from build123d import *

# Parameters (mm, degrees)
SKETCH1_R           = 1.1938
BOSS_EXTRUDE1_DEPTH = 1.5875
SKETCH2_R           = 1.1938
BOSS_EXTRUDE2_DEPTH = 1.5875
BOSS_EXTRUDE3_DEPTH = 3.175
BOSS_EXTRUDE4_DEPTH = 3.175
SKETCH5_W           = 3.656154394
SKETCH5_H           = 41.933387184
CUT_EXTRUDE1_DEPTH  = 78.415745756


with BuildPart() as part:
    # Sketch1 → Boss-Extrude1 (new, symmetric)
    with BuildSketch(Plane(origin=(0, 0, 0), x_dir=(1, 0, 0), z_dir=(0, 1, 0))):
        with BuildLine():
            Line((-40.9956, 2.7686), (40.9956, 2.7686))
            ThreePointArc((40.9956, 2.7686), (43.7642, 0), (40.9956, -2.7686))
            Line((40.9956, -2.7686), (-40.9956, -2.7686))
            ThreePointArc((-40.9956, -2.7686), (-43.7642, 0), (-40.9956, 2.7686))
        make_face()
        with Locations(Location((-40.9956, 0, 0), (0, 0, 270))):
            Circle(SKETCH1_R, mode=Mode.SUBTRACT)
        with Locations(Location((40.9956, 0, 0), (0, 0, 270))):
            Circle(SKETCH1_R, mode=Mode.SUBTRACT)
    extrude(amount=BOSS_EXTRUDE1_DEPTH, both=True)



with BuildPart() as body_2:
    # Sketch2 → Boss-Extrude2 (new, symmetric)
    with BuildSketch(Plane(origin=(0, 0, 0), x_dir=(1, 0, 0), z_dir=(0, 1, 0))):
        with BuildLine():
            Line((-40.9956, -58.2422), (40.9956, -58.2422))
            ThreePointArc((40.9956, -58.2422), (43.7642, -61.0108), (40.9956, -63.7794))
            Line((40.9956, -63.7794), (-40.9956, -63.7794))
            ThreePointArc((-40.9956, -63.7794), (-43.7642, -61.0108), (-40.9956, -58.2422))
        make_face()
        with Locations(Location((-40.9956, -61.0108, 0), (0, 0, 270))):
            Circle(SKETCH2_R, mode=Mode.SUBTRACT)
        with Locations(Location((40.9956, -61.0108, 0), (0, 0, 270))):
            Circle(SKETCH2_R, mode=Mode.SUBTRACT)
    extrude(amount=BOSS_EXTRUDE2_DEPTH, both=True)


with BuildPart() as part_1:
    add(part.part)

    add(body_2.part)  # Boss-Extrude3 merges body 2
    # Sketch3 → Boss-Extrude3 (add)
    with BuildSketch(Plane(origin=(0, 1.5875, 0), x_dir=(1, 0, 0), z_dir=(0, 1, 0))):
        with BuildLine():
            ThreePointArc((-40.9956, -2.7686), (-42.953295834, -1.957695834), (-43.7642, 0))
            Line((-43.7642, 0), (-43.7642, -61.0108))
            ThreePointArc((-43.7642, -61.0108), (-42.953295834, -59.053104166), (-40.9956, -58.2422))
            Line((-40.9956, -58.2422), (-36.444722592, -58.2422))
            Line((-36.444722592, -58.2422), (-36.444722592, -2.7686))
            Line((-36.444722592, -2.7686), (-40.9956, -2.7686))
        make_face()
    extrude(amount=-BOSS_EXTRUDE3_DEPTH)

    # Sketch4 → Boss-Extrude4 (add)
    with BuildSketch(Plane(origin=(0, 1.5875, 0), x_dir=(1, 0, 0), z_dir=(0, 1, 0))):
        with BuildLine():
            ThreePointArc((40.9956, -58.2422), (42.953295834, -59.053104166), (43.7642, -61.0108))
            Line((43.7642, -61.0108), (43.7642, -12.9794))
            Line((43.7642, -12.9794), (34.8742, -12.9794))
            Line((34.8742, -12.9794), (34.8742, -58.2422))
            Line((34.8742, -58.2422), (40.9956, -58.2422))
        make_face()
    extrude(amount=-BOSS_EXTRUDE4_DEPTH)

    # Sketch5 → Cut-Extrude1 (cut, through all)
    with BuildSketch(Plane(origin=(0, 1.5875, 0), x_dir=(1, 0, 0), z_dir=(0, 1, 0))):
        with Locations((41.936122803, -33.946093592)):
            Rectangle(SKETCH5_W, SKETCH5_H)
    extrude(amount=-CUT_EXTRUDE1_DEPTH, mode=Mode.SUBTRACT)


solid = part_1.part
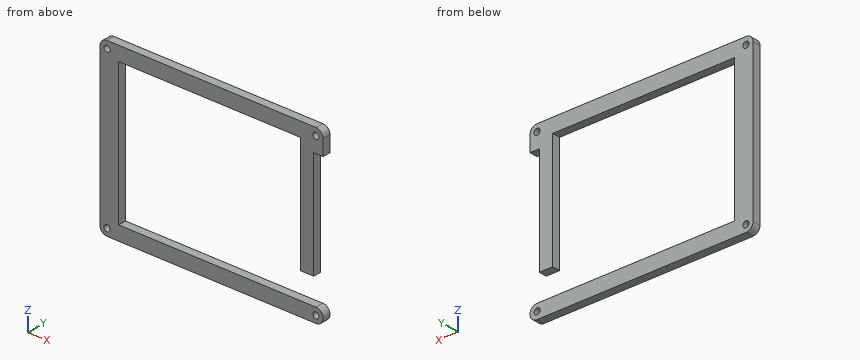
Could you check a few things on this model? Use its own coordinates, in mm. Give positions to 0.01 mm unless a question says otherwise; leave off trailing zeros. Loops run counter-clockwise (first coordinate to the right, second up) from the corner with the lowest first, then second, coordinate; pieces in that order, holes last. Notation, with made-up numbers: (89, -4) -> (144, -4) arc R27 ccw to (144, 30) -> close; hole circle Ø5 at (-16.75, 45). An arc over 180 degrees is marked (long way). Return JSON: item names as keys, results as strings.
Item 1: If we section it at B-B on y = -0.4: List the corners of the cut face in (x, z) for me.
Geometry results:
{"outline": "(-43.76, 0) arc R2.77 ccw to (-41, -2.77) -> (41, -2.77) arc R2.77 ccw to (41, 2.77) -> (-36.44, 2.77) -> (-36.44, 58.24) -> (34.87, 58.24) -> (34.87, 12.98) -> (40.11, 12.98) -> (40.11, 54.91) -> (43.76, 54.91) -> (43.76, 61.01) arc R2.77 ccw to (41, 63.78) -> (-41, 63.78) arc R2.77 ccw to (-43.76, 61.01) -> close; hole circle Ø2.39 at (-41, 0); hole circle Ø2.39 at (-41, 61.01); hole circle Ø2.39 at (41, 0); hole circle Ø2.39 at (41, 61.01)"}
Item 2: I'm going to push flat-ended pins straight in: pin 1 (1 mm diameter, centred on y = -0.5, z = 32.5, fed in from +X); pin 2 (1.6 mm diameter, centred on x = 42, y = 0, fed in from -Z). Where does each tip first touch, or does it pass through?
Geometry results:
{"pin 1": "stops at x = 40.11", "pin 2": "stops at z = -2.76"}
Item 3: I need wall thicknesses on L1, parallel to X at y = 0.7, z = 0; L2, parallel to X at y = 1.45, z = 50.5; L3, parallel to Z at x = -15.5, y = -1.45. Which ranges of each line are inside material? Lowest first, please. Write a range as from..to.
Geometry results:
{"L1": "x = -43.76..-42.19, -39.8..39.8, 42.19..43.76", "L2": "x = -43.76..-36.44, 34.87..40.11", "L3": "z = -2.77..2.77, 58.24..63.78"}
Item 4: If we section it at C-C on x = -15: List the corners of the cut face in (y, z) for me.
Geometry results:
{"outline": "(-1.59, -2.77) -> (1.59, -2.77) -> (1.59, 2.77) -> (-1.59, 2.77) -> close; (-1.59, 58.24) -> (1.59, 58.24) -> (1.59, 63.78) -> (-1.59, 63.78) -> close"}
Item 5: If we section it at A-A on z = 42.5: List the corners of the cut face in (x, y) for me, plus the area to 3 significant figures.
Geometry results:
{"outline": "(-43.76, -1.59) -> (-36.44, -1.59) -> (-36.44, 1.59) -> (-43.76, 1.59) -> close; (34.87, -1.59) -> (40.11, -1.59) -> (40.11, 1.59) -> (34.87, 1.59) -> close", "area": "39.9 mm²"}
